Autodesk Inventor part; units mm, degrees
ref_plane "YZ Plane" through (0, 0, 0) normal (1, 0, 0) x (0, 1, 0)
ref_plane "XZ Plane" through (0, 0, 0) normal (0, 1, 0) x (-1, 0, 0)
ref_plane "XY Plane" through (0, 0, 0) normal (0, 0, 1) x (1, 0, 0)
sketch "Sketch1" plane through (0, 0, 0) normal (0, 1, 0) x (-1, 0, 0)
  line L0 (10.5852, -7.2528) -> (-0.9885, -12.7935)
  line L1 (-0.9885, -12.7935) -> (-11.5737, -5.5406)
  line L2 (-11.5737, -5.5406) -> (-10.5852, 7.2528)
  line L3 (-10.5852, 7.2528) -> (0.9885, 12.7935)
  line L4 (0.9885, 12.7935) -> (11.5737, 5.5406)
  line L5 (11.5737, 5.5406) -> (10.5852, -7.2528)
  point P0 (0, 0)
  point P1 (0, 0)
  dimension "d0" = 22.225
extrude "Extrusion1" add sketch "Sketch1" along normal blind 12.3031
sketch "Sketch2" plane through (0, 12.3031, 0) normal (0, 1, 0) x (1, 0, 0)
  line L0 (-10.5852, 7.2528) -> (-11.5737, -5.5406) construction
  line L1 (11.5737, 5.5406) -> (0.9885, 12.7935) construction
  line L2 (-11.5737, -5.5406) -> (11.5737, 5.5406) construction
  line L3 (10.5852, -7.2528) -> (11.5737, 5.5406) construction
  line L4 (11.5737, 5.5406) -> (10.5852, -7.2528) construction
  line L5 (0.9885, 12.7935) -> (-10.5852, 7.2528) construction
  line L6 (10.5852, -7.2528) -> (-10.5852, 7.2528) construction
  point P0 (0, 0)
hole "Hole1" at (0, 12.3031, 0) direction (0, -1, 0) diameter 10.414 end through all
properties part number "Threaded Rod Nut" material "Aluminum 6061"
Check sheet for the modelled part. Datum: model origin and axes. Units: mm. Coordinates: 2 decimals unless noted, no trailing zeros. Write each loop counter-clockwise with the first axis right and the second up, starting at its lowest first coordinate (ties: lowest second). Pieces come first, ordered by that corner, then holes. Notation, with made-up numbers: M 45.5,79 L 58.5,79 A7 ccw 58.5,90 Z; hole C 84,-1.75 d1. An arc over 180 degrees is marked long. Write item = value, one per line. Start each with the question number.
1. Mould release check, pull along Y, two halves, no side actions. Record for faces 1 (the flat face through (0, 0, -6)), 2 (the flat face through (0, 12.303, -6)), 3 (the flat face through (6.207, 6.065, -9.218)): pulls with the +Y half, pulls with the -Y half, needs draft (parallel to the pull), parting line crosses it, or undercut.
2. Sectioned sample at B-B (y = 10). Record the cut outline in (x, z).
3. Thickness scan on probe 1 along Z at (x, y) = (2.75, 11.75); probe 2 along Z at (x, y) = (-3.5, 7); probe 3 along X at (y, z) = (4.25, -3). Record the ranges inside material, lowest first.
4. Sectioned sample at A-A (z = 0). Record the cut outline in (x, y).
5. Sectioned sample at D-D (x = 8). Record the cut outline in (y, z).
6. Go/stop test with flat-tipped pins: pin 1 (6 mm diameter, centred on x = 0, z = 0, fed in from -Y); pin 2 (2 mm diameter, centred on y = 4.5, z = -9, fed in from +X); pin 3 (1.5 mm diameter, centred on x = -7.5, y = 7, fed in from +Z); pin 4 (5 mm diameter, centred on y = 7.5, z = -0.5, fed in from -X). Record where each tip stops, or that it passes through.
7. Sectioned sample at C-C (x = 0). Record the cut outline in (y, z).
The answers:
q1.face_1 = pulls with the -Y half
q1.face_2 = pulls with the +Y half
q1.face_3 = needs draft
q2.outline = M -11.57,5.54 L -10.59,-7.25 L 0.99,-12.79 L 11.57,-5.54 L 10.59,7.25 L -0.99,12.79 Z; hole C 0,0 d10.41
q3.probe_1 = -11.59 to -4.42, 4.42 to 11
q3.probe_2 = -10.64 to -3.86, 3.86 to 11.07
q3.probe_3 = -10.91 to -4.26, 4.26 to 11.38
q4.outline = M -11.15,0 L -5.21,0 L -5.21,12.3 L -11.15,12.3 Z; M 5.21,0 L 11.15,0 L 11.15,12.3 L 5.21,12.3 Z
q5.outline = M 0,-7.99 L 12.3,-7.99 L 12.3,8.49 L 0,8.49 Z
q6.pin_1 = through
q6.pin_2 = 7.98
q6.pin_3 = 8.85
q6.pin_4 = -11.3
q7.outline = M 0,-12.32 L 12.3,-12.32 L 12.3,-5.21 L 0,-5.21 Z; M 0,5.21 L 12.3,5.21 L 12.3,12.32 L 0,12.32 Z
